For this review, use the dimensioned drawing (mm, ordinates from the lowest corner) and the shaded views. A direction names the side the tool comes from. Coordinates: 2 decimals unless noted, no trailing zeros. Write each loop counter-clockwise with the first axis right and the second up, starting at its lowest first coordinate (ties: lowest second). Pieces come first, ordered by that corner, then holes. Notation, with made-up numbers: M 4.25,-21.75 L 19.25,-21.75 A16 cw 19.25,-8.75 Z; hole C -36,73.25 d8. An arc over 180 degrees is marked long. Return JSON: item names as keys, results as strings. Group by question number.
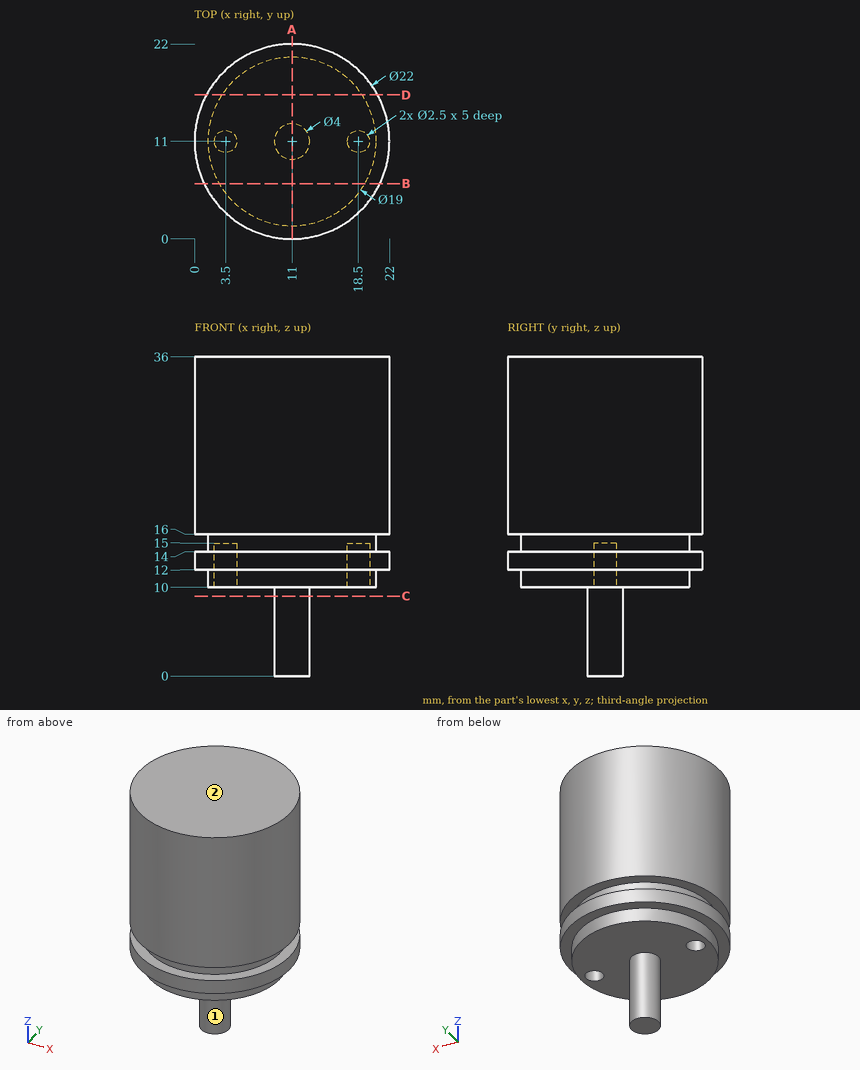
Item 1: Add section D-D (y = 16.25). Write out the cut boundary in (x, z), plus the area to 3 significant figures.
Item 2: Add section B-B (y = 6.25). Write out the cut boundary in (x, z), plus the area to 3 significant figures.
Item 3: Machinability: for the marked faces 1 and 2, which of the approach directions +Z, -Z, +X, -X, +Y, -Y give a long, thin tool a straight path to every point of the face, cutting with its end or side? Answer none if there is none.
Item 4: For pin 1 (1.5 mm diameter, centred on x = 12.5, z = 16.5, fed in from +Y); pin 2 (0.8 mm diameter, centred on x = 18.5, y = 11.5, fed in from -Z); pin 3 (10 mm diameter, centred on x = 19.5, y = 5, fed in from -Z), all flat-tipped, find the tip position at first contact; note any pin that passes through.
Item 5: Add section A-A (x = 11). Write out the cut boundary in (y, z), plus the area to 3 significant figures.
Item 6: Add section C-C (z = 9). Write out the cut boundary in (x, y), plus the area to 3 significant figures.
Item 7: For line 1 (Z direction, x = 8.5, y = 21); line 2 (Z direction, x = 12.25, y = 17.5); line 3 (Y direction, x = 3.5, z = 13.15), list the stretches that pass through material, from the lowest coordinate up.
Geometry check:
{
 "1": {"outline": "M 1.33,12 L 3.08,12 L 3.08,10 L 18.92,10 L 18.92,12 L 20.67,12 L 20.67,14 L 18.92,14 L 18.92,16 L 20.67,16 L 20.67,36 L 1.33,36 L 1.33,16 L 3.08,16 L 3.08,14 L 1.33,14 Z", "area": "489 mm^2"},
 "2": {"outline": "M 1.08,12 L 2.77,12 L 2.77,10 L 19.23,10 L 19.23,12 L 20.92,12 L 20.92,14 L 19.23,14 L 19.23,16 L 20.92,16 L 20.92,36 L 1.08,36 L 1.08,16 L 2.77,16 L 2.77,14 L 1.08,14 Z", "area": "502 mm^2"},
 "3": {"face 1": "-Z", "face 2": "+Z, +X, -X, +Y, -Y"},
 "4": {"pin 1": "y = 21.97", "pin 2": "z = 15", "pin 3": "z = 10"},
 "5": {"outline": "M 0,12 L 1.5,12 L 1.5,10 L 9,10 L 9,0 L 13,0 L 13,10 L 20.5,10 L 20.5,12 L 22,12 L 22,14 L 20.5,14 L 20.5,16 L 22,16 L 22,36 L 0,36 L 0,16 L 1.5,16 L 1.5,14 L 0,14 Z", "area": "600 mm^2"},
 "6": {"outline": "C 11,11 d4", "area": "12.6 mm^2"},
 "7": {"line 1": "12 to 14, 16 to 36", "line 2": "10 to 36", "line 3": "2.95 to 9.75, 12.25 to 19.05"}
}
